Design review of the part built by this model. Coordinates are the model's own, in mm. A direction names the side the tool comes from. Give positions to 0.01 mm unless a question says otherwise; leave off trailing zeros. Loops run counter-clockwise (first coordinate to the right, second up) from the corner with the lowest first, then second, coordinate; pieces in that order, holes last. Notation, with made-up numbers: M 8,2 L 28,2 A20 ccw 28,18 Z; hole C -16.5,74 d3. An arc over 180 degrees is marked long. Answer as CSV lines item,"result".
```python
from build123d import *

# Parameters (mm, degrees)
FASE1_SIZE = 2


with BuildPart() as part:
    # Skizze1 → Rotation1 (revolve)
    with BuildSketch(Plane.XY):
        Polygon((0, 0), (0, 50), (15, 50), (15, 40), (20.322114174, 40), (20.322114174, 38.2), (23.322114174, 38.2), (23.322114174, 40), (30, 40), (30, 0), align=None)
    revolve(axis=Axis((0, 0, 0), (1, 0, 0)))

    # Fase1
    fase1_edges = [part.edges().sort_by_distance(p)[0] for p in [
        (0, -50, 0),
        (30, -40, 0),
    ]]
    chamfer(fase1_edges, length=FASE1_SIZE)


solid = part.part
```
1. For P1, Ø12, axis at x = 19.5, z = -24.5, coming from the -Y side; P2, Ø5, axis at x = 19.5, z = 25, coming from the +Y side; P3, Ø2, axis at x = 10, z = -25.5, coming from the +Y side, all flat-tipped, find the tip position at first contact; note any pin that passes through.
Answer block:
P1,"y = -45.59"
P2,"y = 33.07"
P3,"y = 43.59"
2. To check wall thickness, follow L1, parallel to Y at x = 10.75, z = -1; L2, parallel to X at y = 29, z = -27; L3, parallel to X at y = 46, z = 13. State the ranges of each line that lie inside material, in increasing order. Write a range as [from, to].
Answer block:
L1,"[-49.99, 49.99]"
L2,"[0, 20.32], [23.32, 28.38]"
L3,"[0, 15]"
3. For faces 4 (the flat face through (15, -22, 34)), 5 (the flat face through (23.322, -20.6, -32.4)), 6 (the flat face through (30, -1, 1)), list the 3-axis set-ups (+Z, -Z, +X, -X, +Y, -Y) from which the entire face can be reached by the end or side of a thin tool; tool diameter is ignored.
Answer block:
face 4,"+X"
face 5,"none"
face 6,"+Z, -Z, +X, +Y, -Y"
4. We need section C-C, the plane x = 13.75. Write out the cut boundary in (y, z), plus the area to 3 significant figures.
Answer block:
outline,"C 0,0 d100"
area,"7,850 mm²"
5. The part is to be moulded in two halves that separate along X. For faces 1 (the flat face through (0, 1, 1)), 2 (the cylindrical face through (21.843, -30.314, -23.244)), 3 (the cylindrical face through (8.59, 47.69, 15.02)), say which applies: pulls with the +X half, pulls with the -X half, needs draft (parallel to the pull), parting line crosses it, or undercut.
Answer block:
face 1,"pulls with the -X half"
face 2,"undercut"
face 3,"needs draft"
6. We need section A-A, the plane z = 0. Write out the cut boundary in (x, y).
Answer block:
outline,"M 0,-48 L 2,-50 L 15,-50 L 15,-40 L 20.32,-40 L 20.32,-38.2 L 23.32,-38.2 L 23.32,-40 L 28,-40 L 30,-38 L 30,38 L 28,40 L 23.32,40 L 23.32,38.2 L 20.32,38.2 L 20.32,40 L 15,40 L 15,50 L 2,50 L 0,48 Z"
